Here's the drawing with two shaded views (mm, measured from the low corner). I have some questions. A direction names the side the tool comes from. Give positions to 0.01 mm unless a question says otherwise; leave off trailing zeros. Write each loop counter-clockwise with the first axis right and the second up, starting at its lowest first coordinate (ties: lowest second). Pieces come first, ordered by that corner, then holes. Notation, with made-up numbers: (-19.75, -23.5) - (20.25, -23.5) arc R30 cw to (20.25, 13.5) - close; hole circle Ø8 at (23.25, 56.5). An arc over 180 degrees is marked (long way). Use one line per item in the form item = value.
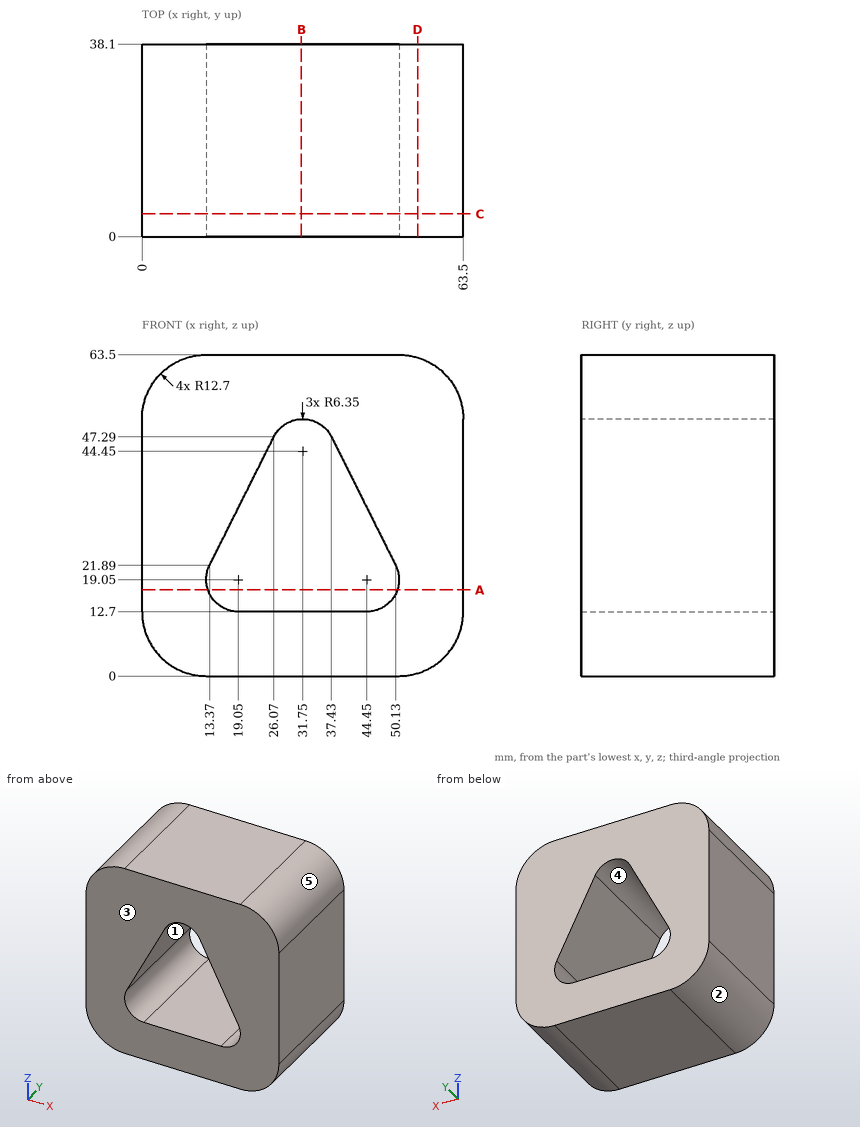
1. Imagine slicing it at B-B, the plane x = 31.5. List the corners of the cut face in (y, z) for me (1 decimal).
Response values:
outline = (0, 0) - (38.1, 0) - (38.1, 12.7) - (0, 12.7) - close; (0, 50.8) - (38.1, 50.8) - (38.1, 63.5) - (0, 63.5) - close
2. For pin 1 (1 mm diameter, centred on x = 45, z = 28.5, fed in from -Y), with a flat end and sliding along its axis, tell me the tip position at first contact or that it passes through.
Response values:
pin_1 = through
3. Imagine slicing it at D-D, the plane x = 54.5. List the corners of the cut face in (y, z) for me.
Response values:
outline = (0, 0.55) - (38.1, 0.55) - (38.1, 62.95) - (0, 62.95) - close
4. If I drill on line 1 (X direction, y = 30.5, z = 19.5); line 2 (X direction, y = 23.5, z = 33) (1 decimal); line 3 (Z direction, x = 39.5, y = 22), over which ranges is the centre line in solid material (lowest first)? Write a range as from..to.
Response values:
line_1 = 0..12.72, 50.78..63.5
line_2 = 0..18.9, 44.6..63.5
line_3 = 0..12.7, 43.15..63.5
5. If we mould it in two halves opening along Z, with no side actions, what happens to the marked faces 1, 2 and 3? For each: pulls with the +Z half, pulls with the -Z half, needs draft (parallel to the pull), parting line crosses it, or undercut.
Response values:
face_1 = undercut
face_2 = pulls with the -Z half
face_3 = needs draft
6. Which directions (+Z, -Z, +X, -X, +Y, -Y) give clear straight access to the entire face, cutting with the end or side of a thin tool? Please do the marked faces 4 and 5.
Response values:
face_4 = +Y, -Y
face_5 = +Z, +X, +Y, -Y
7. Imagine slicing it at C-C, the plane y = 4.5. List the corners of the cut face in (x, z) for me, and give its area (3 significant figures).
Response values:
outline = (0, 12.7) arc R12.7 ccw to (12.7, 0) - (50.8, 0) arc R12.7 ccw to (63.5, 12.7) - (63.5, 50.8) arc R12.7 ccw to (50.8, 63.5) - (12.7, 63.5) arc R12.7 ccw to (0, 50.8) - close; hole (13.37, 21.89) arc R6.35 ccw to (19.05, 12.7) - (44.45, 12.7) arc R6.35 ccw to (50.13, 21.89) - (37.43, 47.29) arc R6.35 ccw to (26.07, 47.29) - close
area = 2,920 mm²
8. Imagine slicing it at A-A, the plane z = 17. List the corners of the cut face in (x, y) for me.
Response values:
outline = (0, 0) - (13.04, 0) - (13.04, 38.1) - (0, 38.1) - close; (50.46, 0) - (63.5, 0) - (63.5, 38.1) - (50.46, 38.1) - close
